from build123d import *

# Parameters (mm, degrees)
SALIENTE_EXTRUIR1_DEPTH                              = 7
SALIENTE_EXTRUIR1_DEPTH_BACK                         = 7
CROQUIS1_R                                           = 4
TALADRO_DE_MARGEN_PARA_M51_D                         = 5.5
CORTAR_EXTRUIR1_DEPTH                                = 40.570696228
CORTAR_EXTRUIR1_DEPTH_BACK                           = 40.570696228
CROQUIS6_W                                           = 1
CROQUIS6_H                                           = 17.84861806
REFRENTADO_PARA_TORNILLO_CON_CABEZA_HUEC_D           = 4.5
REFRENTADO_PARA_TORNILLO_CON_CABEZA_HUEC_CBORE_D     = 8
REFRENTADO_PARA_TORNILLO_CON_CABEZA_HUEC_CBORE_DEPTH = 4.4


with BuildPart() as part:
    # Croquis1 → Saliente-Extruir1 (new, two sides: drawn at the far end of the back side and taken through both)
    with BuildSketch(Plane.XY.offset(-SALIENTE_EXTRUIR1_DEPTH_BACK)):
        Polygon((-21, 0), (21, 0), (21, 6), (9, 6), (9, 32.8), (-9, 32.8), (-9, 6), (-21, 6), align=None)
        with Locations((0, 20)):
            Circle(CROQUIS1_R, mode=Mode.SUBTRACT)
    extrude(amount=SALIENTE_EXTRUIR1_DEPTH + SALIENTE_EXTRUIR1_DEPTH_BACK)

    # Taladro de margen para M51 (through all)
    with Locations(Plane(origin=(0, 0, 0), x_dir=(-1, 0, 0), z_dir=(0, -1, 0))):
        with Locations((-16, 0), (16, 0)):
            Hole(TALADRO_DE_MARGEN_PARA_M51_D / 2)

    # Croquis6 → Cortar-Extruir1 (cut, two sides: drawn at the far end of the back side and taken through both)
    with BuildSketch(Plane.XY.offset(-CORTAR_EXTRUIR1_DEPTH_BACK)):
        with Locations((0, 28.92430903)):
            Rectangle(CROQUIS6_W, CROQUIS6_H)
    extrude(amount=CORTAR_EXTRUIR1_DEPTH + CORTAR_EXTRUIR1_DEPTH_BACK, mode=Mode.SUBTRACT)

    # Refrentado para tornillo con cabeza hueca de M41 (through all)
    with Locations(Plane(origin=(9, 0, 0), x_dir=(0, 0, -1), z_dir=(1, 0, 0))):
        with Locations((0, 27.8)):
            CounterBoreHole(REFRENTADO_PARA_TORNILLO_CON_CABEZA_HUEC_D / 2, REFRENTADO_PARA_TORNILLO_CON_CABEZA_HUEC_CBORE_D / 2, REFRENTADO_PARA_TORNILLO_CON_CABEZA_HUEC_CBORE_DEPTH)


solid = part.part
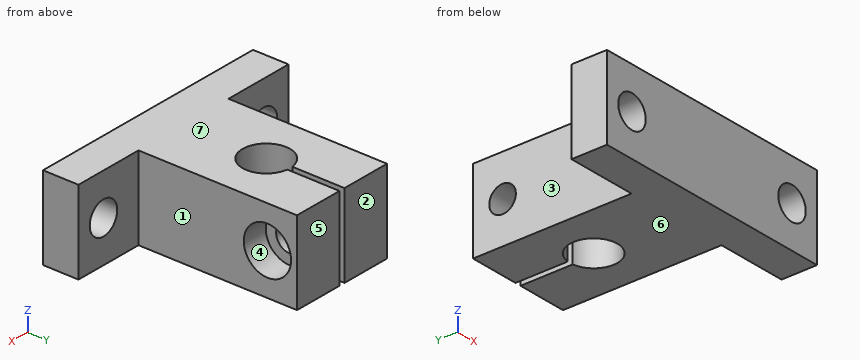
Design review of the part built by this model. Coordinates are the model's own, in mm. Face numbers are marked on the shaded views. A direction names the side the tool comes from. Round coordinates to 2 decimals unless told otherwise and drop trailing zeros. Order: outer loops, then holes, each group sorted by start corner. A loop starts at its lowest first (then second) coordinate and runs counter-clockwise, first axis right, second up.
1) Consider section C-C (x = -16). State the section outline as (y, z) points, plus the area to 3 significant figures.
The answers:
outline: (0, -7) - (6, -7) - (6, -2.75) - (0, -2.75) - close; (0, 2.75) - (6, 2.75) - (6, 7) - (0, 7) - close
area: 51.0 mm2
2) Consider section A-A (y = 27.8). State the section outline as (x, z) points.
The answers:
outline: (-9, -7) - (-0.5, -7) - (-0.5, -2.25) - (-9, -2.25) - close; (-9, 2.25) - (-0.5, 2.25) - (-0.5, 7) - (-9, 7) - close; (0.5, -7) - (9, -7) - (9, -4) - (4.6, -4) - (4.6, -2.25) - (0.5, -2.25) - close; (0.5, 2.25) - (4.6, 2.25) - (4.6, 4) - (9, 4) - (9, 7) - (0.5, 7) - close
3) Machinability: for the marked faces 1, 2 and 3, which of the approach directions +Z, -Z, +X, -X, +Y, -Y give a long, thin tool a straight path to every point of the face, cutting with its end or side? Answer none if there is none.
The answers:
face 1: +Z, -Z, +X, +Y
face 2: +Z, -Z, +X, -X, +Y
face 3: +Z, -Z, -X, +Y
4) Draft analysis for pull direction Z (two halves, no side actions). For the marked faces 4, 5, 6 and 7, state which applies: released by +Z, released by -Z, zero draft, split by the parting line, or undercut.
The answers:
face 4: undercut
face 5: zero draft
face 6: released by -Z
face 7: released by +Z
5) For L1, parallel to Y at x = -7, z = 0; L2, parallel to Z at x = 16, y = 1; L3, parallel to Y at x = 3.6, z = 0, list the stretches that pass through material, from the lowest coordinate up.
The answers:
L1: y = 0 to 25.55, 30.05 to 32.8
L2: z = -7 to -2.75, 2.75 to 7
L3: y = 0 to 18.26, 21.74 to 25.55, 30.05 to 32.8
6) Clearance check with flat-ended pins moving along their axes: pin 1 Ø6 at (x, z) = (16.5, 3.5) entering from +Y; pin 2 Ø4.5 at (y, z) = (30, 3) entering from -X; pin 3 Ø2.5 at (y, z) = (27.8, 0) entering from -X; pin 4 Ø4 at (y, z) = (29, -1.5) entering from +X. State where each tip first meets the part, or that it passes through.
The answers:
pin 1: stops at y = 6
pin 2: stops at x = -9
pin 3: passes through
pin 4: stops at x = 4.6
7) Consider section B-B (z = 0). Count the separate pieces of the cut face and the enclosed holes in it, plus the area to 3 significant figures.
The answers:
separate pieces: 5
enclosed holes: 0
area: 517 mm2
8) Consider section D-D (x = -1). State the section outline as (y, z) points.
The answers:
outline: (0, -7) - (16.13, -7) - (16.13, 7) - (0, 7) - close; (23.87, -7) - (32.8, -7) - (32.8, 7) - (23.87, 7) - close; hole circle Ø4.5 at (27.8, 0)
